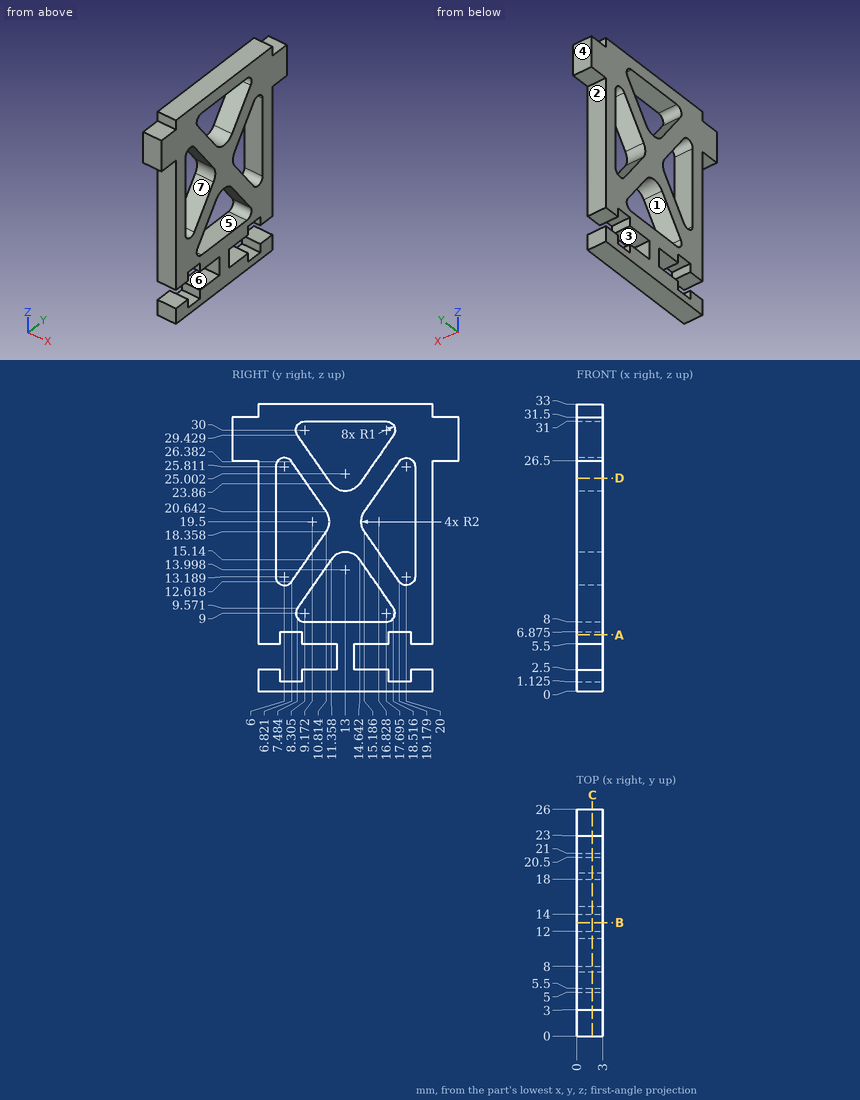
The drawing under review shows one solid part. Ordinate dimensions are in mm from its lowest x, y, z. A direction names the side the tool comes from. Give positions to 0.01 mm unless a question says otherwise; leave off trailing zeros. Loops run counter-clockwise (first coordinate to the right, second up) from the corner with the lowest first, then second, coordinate; pieces in that order, holes last. Notation, with made-up numbers: M -12,-20 L 10,-20 A21 cw 10,9 Z; hole C 87.25,14 d4. An arc over 180 degrees is marked long. Return JSON: item names as keys, results as strings. Group by question number.
Item 1: For probe 1 along Z at (x, y) = (1.85, 20) (1 decimal); probe 2 along Y at (x, z) = (1.85, 19.5); probe 3 along Z at (x, y) = (0.8, 22.5), list the stretches that pass through material, from the lowest coordinate up.
Item 2: We need section D-D (z = 24.5). Give the boundary of the cut face in (x, y), and give its area (3 significant figures).
Item 3: Tool access review of the marked faces 1, 2 and 3: name each direction out of +Z, -Z, +X, -X, +Y, -Y from which nothing blocks a thin tool from reaching the whole face with its end or side.
Item 4: Mouldability with a two-part tool opening along Y and no side actions: class the marked faces 4, 5, 6 and 7 as released by +Y, released by -Y, zero draft, split by the parting line, or undercut.
Item 5: We need section C-C (x = 1.8). Give the number of separate pieces and of enclosed holes in the cut face.
Item 6: We need section A-A (z = 6.5). Give the boundary of the cut face in (x, y), and give its area (3 significant figures).
Item 7: We need section B-B (y = 13). Give the boundary of the cut face in (x, z).
Item 8: Insertion check: pin 1 Ø1.1 at (x, z) = (1.5, 6.5) entering from +Y; pin 2 Ø0.9 at (x, y) = (2, 24) entering from -Z; pin 3 Ø1.2 at (x, z) = (1, 32.5) entering from -Y. Each pin has a flat end and moves straight along its axis. Give the tip position at first contact, or say it passes through.
Output:
{
 "1": {"probe 1": "z = 0 to 1.1, 6.9 to 12.2, 26.8 to 33", "probe 2": "y = 3 to 5, 11.17 to 14.83, 21 to 23", "probe 3": "z = 0 to 2.5, 5.5 to 33"},
 "2": {"outline": "M 0,3 L 3,3 L 3,5 L 0,5 Z; M 0,8.13 L 3,8.13 L 3,10.91 L 0,10.91 Z; M 0,15.09 L 3,15.09 L 3,17.87 L 0,17.87 Z; M 0,21 L 3,21 L 3,23 L 0,23 Z", "area": "28.7 mm^2"},
 "3": {"face 1": "+X, -X", "face 2": "-Z, +X, -X, +Y", "face 3": "+X, -X, +Y"},
 "4": {"face 4": "released by +Y", "face 5": "undercut", "face 6": "zero draft", "face 7": "undercut"},
 "5": {"separate pieces": "1", "enclosed holes": "4"},
 "6": {"outline": "M 0,3 L 3,3 L 3,5.5 L 0,5.5 Z; M 0,8 L 3,8 L 3,18 L 0,18 Z; M 0,20.5 L 3,20.5 L 3,23 L 0,23 Z", "area": "45.0 mm^2"},
 "7": {"outline": "M 0,0 L 3,0 L 3,8 L 0,8 Z; M 0,16 L 3,16 L 3,23 L 0,23 Z; M 0,31 L 3,31 L 3,33 L 0,33 Z"},
 "8": {"pin 1": "stops at y = 23", "pin 2": "stops at z = 26.5", "pin 3": "stops at y = 3"}
}
